```python
from build123d import *

# Parameters (mm, degrees)
SKETCH1_W           = 25.4
SKETCH1_H           = 50.8
SKETCH1_W_2         = 20.32
SKETCH1_H_2         = 45.72
EXTRUDE_THIN1_DEPTH = 152.4
SKETCH2_R           = 1.5875
CUT_EXTRUDE1_DEPTH  = 51.8
LPATTERN1_COUNT     = 50
LPATTERN1_PITCH     = 25.4


with BuildPart() as part:
    # Sketch1 → Extrude-Thin1 (new body)
    with BuildSketch(Plane.XY):
        with Locations((12.7, 25.4)):
            Rectangle(SKETCH1_W, SKETCH1_H)
        with Locations((12.7, 25.4)):
            Rectangle(SKETCH1_W_2, SKETCH1_H_2, mode=Mode.SUBTRACT)
    extrude(amount=EXTRUDE_THIN1_DEPTH)

    # Sketch2 → Cut-Extrude1 (cut, through all)
    with BuildSketch(Plane(origin=(0, 50.8, 0), x_dir=(1, 0, 0), z_dir=(0, 1, 0))):
        with Locations((12.7, -136.525)):
            Circle(SKETCH2_R)
    cut_extrude1 = extrude(amount=-CUT_EXTRUDE1_DEPTH, mode=Mode.SUBTRACT)

    # LPattern1: Cut-Extrude1 ×50
    with Locations(*[(0, 0, -i * LPATTERN1_PITCH) for i in range(1, LPATTERN1_COUNT)]):
        add(cut_extrude1, mode=Mode.SUBTRACT)


solid = part.part
```
Could you check a few things on this model? Use its own coordinates, in mm. A direction names the side the tool comes from. Give positions to 0.01 mm unless a question says otherwise; leave off trailing zeros. Order: outer loops, then holes, each group sorted by start corner. A loop starts at its lowest first (then second) coordinate and runs counter-clockwise, first axis right, second up.
Q1. If I drill on line 1 along Y through (x, z) = (10.5, 89); line 2 along X through (y, z) = (34.5, 67), over which ranges is the centre line in solid material (lowest first)?
Q2. For faces 1 (the flat face through (2.54, 25, 75)), 2 (the cylindrical face through (13.433, 1.288, 36.333)), which set-ups out of +Z, -Z, +X, -X, +Y, -Y let a thin tool reach every point of the face, with its end or its side?
Q3. Suppose I cut it at A-A, the plane x = 18.75. Write out the boundary of the cut face in (y, z), and give its area (3 significant figures).
Q4. We'd pull the mould along Y, two halves only. Please class faces 3 (the flat face through (13, 0, 75)), 4 (the flat face through (2, 27, 0)), 5 (the flat face through (22.86, 25, 75)): +Y half, -Y half, draft (parallel to the pull), parting line (faces both ways), or undercut.
Q5. I'm going to push flat-ended pins straight in: P1, Ø3.5, axis at x = 12.7, z = 85.725, coming from the -Y side; P2, Ø1.9, axis at x = 12.7, z = 60.325, coming from the +Y side (1 decimal). Where does each tip first touch, or does it pass through?
Q6. Suppose I cut it at B-B, the plane y = 19. Write out the boundary of the cut face in (x, z), and give its area (3 significant figures).
Q7. Suppose I cut it at D-D, the plane x = 12.7. Count the separate pieces of the cut face and the enclosed holes in it, and give its area (3 significant figures).
Q8. Suppose I cut it at C-C, the plane z = 94. Write out the boundary of the cut face in (x, y), and give its area (3 significant figures).
Solution:
1. line 1: y = 0 to 2.54, 48.26 to 50.8
1. line 2: x = 0 to 2.54, 22.86 to 25.4
2. face 1: +Z, -Z
2. face 2: +Y, -Y
3. outline: (0, 0) - (2.54, 0) - (2.54, 152.4) - (0, 152.4) - close; (48.26, 0) - (50.8, 0) - (50.8, 152.4) - (48.26, 152.4) - close
3. area: 774 mm2
4. face 3: -Y half
4. face 4: draft
4. face 5: undercut
5. P1: stops at y = 0
5. P2: passes through
6. outline: (0, 0) - (2.54, 0) - (2.54, 152.4) - (0, 152.4) - close; (22.86, 0) - (25.4, 0) - (25.4, 152.4) - (22.86, 152.4) - close
6. area: 774 mm2
7. separate pieces: 14
7. enclosed holes: 0
7. area: 677 mm2
8. outline: (0, 0) - (25.4, 0) - (25.4, 50.8) - (0, 50.8) - close; hole (2.54, 2.54) - (22.86, 2.54) - (22.86, 48.26) - (2.54, 48.26) - close
8. area: 361 mm2
